The listing builds one solid part. Answer for the finished solid, in the listing's coordinates (mm). A direction names the side the tool comes from. Round coordinates to 2 decimals unless told otherwise and drop trailing zeros.
(1) A cutting plane is placed at A-A, the plane y = -195. Give the number of separate pieces and of enclosed holes in the cut face, and give its area (3 significant figures).
(2) Find the intervals of material crossed by probe 1 along Z at (x, y) = (0, 223.5); probe 2 along Z at (x, y) = (13, 434); probe 3 along Z at (x, y) = (-10.25, -422), in increasing order.
(3) For faces 1 (the face through (4, -7, 0)), 2 (the face through (-15, -7, 0)), determine the directions among +Z, -Z, +X, -X, +Y, -Y from which every point of the face is accessible in a straight line to the end or side of a thin tool.
(4) Each of these flat-tipped pins is pushed along its axis until it touches: pin 1 Ø6.5 at (y, z) = (61.5, 16.5) entering from +X; pin 2 Ø2.5 at (x, y) = (0.5, 146.5) entering from -Z; pin 3 Ø2.5 at (x, y) = (-2, -20.5) entering from +Z. Where does it stop, or does it pass through?
(5) The mould has two halves that part along Z. Classify faces 3 (the face through (-7, -500, 0)), 4 (the face through (-4, -7, 0)): +Z half, -Z half, draft (parallel to the pull), parting line (faces both ways), or undercut.
from build123d import *

# Parameters (mm, degrees)
F1_DEPTH = 500
F2_R     = 3.4
F2_W     = 8
F2_H     = 20
F3_DEPTH = 1000
F4_R     = 3


with BuildPart() as f1:
    # F0 (on Front) → F1 (new body, symmetric)
    with BuildSketch(Plane.XZ):
        Polygon((15, 19), (15, 30), (4, 30), (4, 20), (-4, 20), (-4, 30), (-15, 30), (-15, 19), (-5, 19), (-5, 11), (-15, 11), (-15, -11), (-5, -11), (-5, -19), (-15, -19), (-15, -30), (-4, -30), (-4, -20), (4, -20), (4, -30), (15, -30), (15, -19), (5, -19), (5, -11), (15, -11), (15, 11), (5, 11), (5, 19), align=None)
    extrude(amount=F1_DEPTH, both=True)

    # F2 (on face) → F3 (cut)
    with BuildSketch(Plane.XZ.offset(500)):
        with Locations((0, -15)):
            Circle(F2_R)
        Rectangle(F2_W, F2_H)
        with Locations((0, 15)):
            Circle(F2_R)
    extrude(amount=-F3_DEPTH, mode=Mode.SUBTRACT)

    # F4
    f4_edges = [f1.edges().sort_by_distance(p)[0] for p in [
        (-15, 0, -30),
        (15, 0, -30),
        (15, 0, 30),
        (-15, 0, 30),
    ]]
    fillet(f4_edges, radius=F4_R)


solid = f1.part
Solutions:
1. separate pieces: 1
1. enclosed holes: 3
1. area: 1,080 mm2
2. probe 1: z = -20 to -18.4, -11.6 to -10, 10 to 11.6, 18.4 to 20
2. probe 2: z = -29.83 to -19, -11 to 11, 19 to 29.83
2. probe 3: z = -30 to -19, -11 to 11, 19 to 30
3. face 1: +Y, -Y
3. face 2: +Z, -Z, -X, +Y, -Y
4. pin 1: stops at x = 15
4. pin 2: stops at z = -20
4. pin 3: stops at z = 20
5. face 3: draft
5. face 4: undercut
